from build123d import *

# Parameters (mm, degrees)
SKETCH1_W           = 150
SKETCH1_H           = 150
SKETCH1_W_2         = 140
SKETCH1_H_2         = 140
BOSS_EXTRUDE1_DEPTH = 90
SKETCH2_W           = 150
SKETCH2_H           = 150
BOSS_EXTRUDE2_DEPTH = 4
SKETCH3_W           = 140
SKETCH3_H           = 140
SKETCH3_R           = 12.5
BOSS_EXTRUDE3_DEPTH = 10
FILLET1_R           = 5


with BuildPart() as part:
    # Sketch1 → Boss-Extrude1 (new body)
    with BuildSketch(Plane(origin=(0, 0, 0), x_dir=(1, 0, 0), z_dir=(0, 1, 0))):
        with Locations((70, 70)):
            Rectangle(SKETCH1_W, SKETCH1_H)
        with Locations((70, 70)):
            Rectangle(SKETCH1_W_2, SKETCH1_H_2, mode=Mode.SUBTRACT)
    extrude(amount=BOSS_EXTRUDE1_DEPTH)

    # Sketch2 → Boss-Extrude2 (add)
    with BuildSketch(Plane.XZ):
        with Locations((70, -70)):
            Rectangle(SKETCH2_W, SKETCH2_H)
    extrude(amount=BOSS_EXTRUDE2_DEPTH)

    # Sketch3 → Boss-Extrude3 (add)
    with BuildSketch(Plane(origin=(0, 0, 0), x_dir=(1, 0, 0), z_dir=(0, 1, 0))):
        with Locations((70, 70)):
            Rectangle(SKETCH3_W, SKETCH3_H)
        with Locations(Location((17.5, 17.5, 0), (0, 0, 270))):
            Circle(SKETCH3_R, mode=Mode.SUBTRACT)
        with Locations(Location((17.5, 52.5, 0), (0, 0, 270))):
            Circle(SKETCH3_R, mode=Mode.SUBTRACT)
        with Locations(Location((17.5, 87.5, 0), (0, 0, 270))):
            Circle(SKETCH3_R, mode=Mode.SUBTRACT)
        with Locations(Location((122.5, 17.5, 0), (0, 0, 270))):
            Circle(SKETCH3_R, mode=Mode.SUBTRACT)
        with Locations(Location((87.5, 17.5, 0), (0, 0, 270))):
            Circle(SKETCH3_R, mode=Mode.SUBTRACT)
        with Locations(Location((52.5, 17.5, 0), (0, 0, 270))):
            Circle(SKETCH3_R, mode=Mode.SUBTRACT)
        with Locations(Location((122.5, 52.5, 0), (0, 0, 270))):
            Circle(SKETCH3_R, mode=Mode.SUBTRACT)
        with Locations(Location((87.5, 52.5, 0), (0, 0, 270))):
            Circle(SKETCH3_R, mode=Mode.SUBTRACT)
        with Locations(Location((52.5, 52.5, 0), (0, 0, 270))):
            Circle(SKETCH3_R, mode=Mode.SUBTRACT)
        with Locations(Location((122.5, 87.5, 0), (0, 0, 270))):
            Circle(SKETCH3_R, mode=Mode.SUBTRACT)
        with Locations(Location((87.5, 87.5, 0), (0, 0, 270))):
            Circle(SKETCH3_R, mode=Mode.SUBTRACT)
        with Locations(Location((52.5, 87.5, 0), (0, 0, 270))):
            Circle(SKETCH3_R, mode=Mode.SUBTRACT)
        with Locations(Location((122.5, 122.5, 0), (0, 0, 270))):
            Circle(SKETCH3_R, mode=Mode.SUBTRACT)
        with Locations(Location((87.5, 122.5, 0), (0, 0, 270))):
            Circle(SKETCH3_R, mode=Mode.SUBTRACT)
        with Locations(Location((52.5, 122.5, 0), (0, 0, 270))):
            Circle(SKETCH3_R, mode=Mode.SUBTRACT)
        with Locations(Location((17.5, 122.5, 0), (0, 0, 270))):
            Circle(SKETCH3_R, mode=Mode.SUBTRACT)
    extrude(amount=BOSS_EXTRUDE3_DEPTH)

    # Fillet1
    fillet1_edges = [part.edges().sort_by_distance(p)[0] for p in [
        (145, -4, -70),
        (70, -4, 5),
        (-5, -4, -70),
        (70, -4, -145),
        (-5, 43, -145),
        (145, 43, -145),
        (145, 43, 5),
        (-5, 43, 5),
    ]]
    fillet(fillet1_edges, radius=FILLET1_R)


solid = part.part
Here's how the part is built. I have some questions about the finished solid (model axes, mm). A direction names the side the tool comes from. Give positions to 0.01 mm unless a question says otherwise; leave off trailing zeros. Order: outer loops, then holes, each group sorted by start corner. A loop starts at its lowest first (then second) coordinate and runs counter-clockwise, first axis right, second up. Notation, with made-up numbers: (29.5, 69) -> (88.5, 69) arc R26 ccw to (88.5, 101) -> close; hole circle Ø2 at (27.25, 58). An arc over 180 degrees is marked (long way). One line per item, written item: value. Start each with the question number.
1. We'd pull the mould along Z, two halves only. Please class faces 1 (the face through (17, 0, -52)), 2 (the face through (143, 46, 4)), 3 (the face through (-5, 46, -71)), 4 (the face through (17, 0, -122)): released by +Z, released by -Z, zero draft, split by the parting line, or undercut.
2. Imagine slicing it at A-A, the plane y = 21. List the corners of the cut face in (x, z) for me, plus the area to 3 significant figures.
3. Imagine slicing it at B-B, the plane z = -52.5. List the corners of the cut face in (x, y) for me, plus the area to 3 significant figures.
4. I need wall thicknesses on probe 1 along X at (y, z) = (4, -17); probe 2 along Z at (x, y) = (87, 3); probe 3 along X at (y, z) = (68, -87). Which ranges of each line are inside material? Lowest first, please. Write a range as from..to.
5. For faces 5 (the face through (-4, 45, -143)), 6 (the face through (0, 49, -69)), which set-ups out of +Z, -Z, +X, -X, +Y, -Y let a thin tool reach every point of the face, with its end or its side?
6. Imagine slicing it at C-C, the plane x = 122.5. List the corners of the cut face in (y, z) for me, plus the area to 3 significant figures.
7. Will these pins go through, and if not, where does the flat tip stop? pin 1 Ø1.5 at (x, z) = (11, -92.5) entering from +Y; pin 2 Ø12 at (x, z) = (32.5, -77.5) entering from +Y.
Values follow:
1. face 1: undercut
1. face 2: released by +Z
1. face 3: zero draft
1. face 4: undercut
2. outline: (-5, -140) arc R5 ccw to (0, -145) -> (140, -145) arc R5 ccw to (145, -140) -> (145, 0) arc R5 ccw to (140, 5) -> (0, 5) arc R5 ccw to (-5, 0) -> close; hole (0, -140) -> (140, -140) -> (140, 0) -> (0, 0) -> close
2. area: 2,880 mm2
3. outline: (-5, 1) arc R5 ccw to (0, -4) -> (140, -4) arc R5 ccw to (145, 1) -> (145, 90) -> (140, 90) -> (140, 10) -> (135, 10) -> (135, 0) -> (110, 0) -> (110, 10) -> (100, 10) -> (100, 0) -> (75, 0) -> (75, 10) -> (65, 10) -> (65, 0) -> (40, 0) -> (40, 10) -> (30, 10) -> (30, 0) -> (5, 0) -> (5, 10) -> (0, 10) -> (0, 90) -> (-5, 90) -> close
3. area: 1,890 mm2
4. probe 1: x = -5..5.01, 29.99..40.01, 64.99..75.01, 99.99..110.01, 134.99..145
4. probe 2: z = -145..-134.99, -110.01..-99.99, -75.01..-64.99, -40.01..-29.99, -5.01..5
4. probe 3: x = -5..0, 140..145
5. face 5: -Z, -X, +Y, -Y
5. face 6: +Y
6. outline: (-4, -140) arc R5 ccw to (1, -145) -> (90, -145) -> (90, -140) -> (10, -140) -> (10, -135) -> (0, -135) -> (0, -110) -> (10, -110) -> (10, -100) -> (0, -100) -> (0, -75) -> (10, -75) -> (10, -65) -> (0, -65) -> (0, -40) -> (10, -40) -> (10, -30) -> (0, -30) -> (0, -5) -> (10, -5) -> (10, 0) -> (90, 0) -> (90, 5) -> (1, 5) arc R5 ccw to (-4, 0) -> close
6. area: 1,890 mm2
7. pin 1: stops at y = 0
7. pin 2: stops at y = 10
